Autodesk Inventor part; units mm, degrees
ref_plane "YZ Plane" through (0, 0, 0) normal (1, 0, 0) x (0, 1, 0)
ref_plane "XZ Plane" through (0, 0, 0) normal (0, 1, 0) x (-1, 0, 0)
ref_plane "XY Plane" through (0, 0, 0) normal (0, 0, 1) x (1, 0, 0)
ref_plane "Work Plane1" through (0, 0, 0) normal (0, 0, 1) x (1, 0, 0)
sketch "Sketch1" plane through (0, 0, 0) normal (0, 0, 1) x (1, 0, 0)
  circle A0 centre (0, 55.5) radius 2
  circle A1 centre (55.5, 0) radius 2
  circle A2 centre (-55.5, 0) radius 2
  circle A3 centre (0, -55.5) radius 2
  circle A4 centre (-39.2444, -39.2444) radius 4
  circle A5 centre (39.2444, -39.2444) radius 4
  circle A6 centre (-39.2444, 39.2444) radius 4
  circle A7 centre (39.2444, 39.2444) radius 4
  circle A8 centre (0, 0) radius 61.5
  circle A9 centre (0, 0) radius 49.5
  circle A10 centre (0, 0) radius 75
  line L0 (106.066, 0) -> (0, -106.066)
  line L1 (0, -55.5) -> (-55.5, 0) construction
  line L2 (106.066, 0) -> (53.033, 53.033)
  line L3 (0, -106.066) -> (-53.033, -53.033)
  point P0 (0, 0)
  dimension "d0" = 150
extrude "Extrusion1" add sketch "Sketch1" along normal blind 6.35 contours A4 | A5 | A6 | A7 | A8 | A10 | A10 L2 L0 | L0 L3 A10
properties part number "AxisBoard"
Geometry: final body of the model. Coordinates: model frame, mm. Give positions to 0.01 mm unless a question says otherwise; leave off trailing zeros. Order: outer loops, then holes, each group sorted by start corner. A loop starts at its lowest first (then second) coordinate and runs counter-clockwise, first axis right, second up. Notation, with made-up numbers: (42.25, -34.75) -> (85.25, -34.75) arc R31 cw to (85.25, -9.75) -> close; hole circle Ø7 at (80.25, 18). An arc over 180 degrees is marked (long way). Put each result on its own line as item: value.
Q1. Draft query along X for faces 1 (the face through (-57.498, -0.088, 3.131)), 2 (the face through (-26.145, -79.921, 3.131)), 3 (the face through (53.502, -0.088, 3.131)), 4 (the face through (53.775, -52.291, 3.131)). Return one class per face: released by +X, released by -X, zero draft, split by the parting line, or undercut.
Here are the results:
face 1: undercut
face 2: released by -X
face 3: undercut
face 4: released by +X
Q2. Section A-A, the plane y = 28. Return loops of the section in (x, z).
Here are the results:
outline: (-69.58, 0) -> (-40.82, 0) -> (-40.82, 6.35) -> (-69.58, 6.35) -> close; (40.82, 0) -> (78.07, 0) -> (78.07, 6.35) -> (40.82, 6.35) -> close
Q3. Section C-C, the plane x = -38.5. Return loops of the section in (y, z), then the cut area to 3 significant figures.
Here are the results:
outline: (-67.57, 0) -> (-31.11, 0) -> (-31.11, 6.35) -> (-67.57, 6.35) -> close; (31.11, 0) -> (64.36, 0) -> (64.36, 6.35) -> (31.11, 6.35) -> close
area: 443 mm^2
Q4. Pin query (flat end, axial travel): pin 1 (6 mm diameter, centred on x = 31.5, y = -66, fed in from -Z); pin 2 (2 mm diameter, centred on x = -23.5, z = 1.5, fed in from -Y). Return the tip coordinate at first contact, or that it passes through.
Here are the results:
pin 1: stops at z = 0
pin 2: stops at y = -83.57
Q5. Material intervals for L1, parallel to Y at x = 0, z = 2.25; L2, parallel to Y at x = -34, z = 4; L3, parallel to Y at x = -9, z = 4.5, sorted ascending.
Here are the results:
L1: y = -106.07 to -57.5, -53.5 to -49.5, 49.5 to 53.5, 57.5 to 75
L2: y = -72.07 to -35.98, 35.98 to 66.85
L3: y = -97.07 to -48.67, 48.67 to 74.46
Q6. Section D-D, the plane x = 82.5. Return loops of the section in (y, z), then the cut area to 3 significant figures.
Here are the results:
outline: (-23.57, 0) -> (23.57, 0) -> (23.57, 6.35) -> (-23.57, 6.35) -> close
area: 299 mm^2
